from build123d import *

# Parameters (mm, degrees)
SKETCH1_W           = 25.4
SKETCH1_H           = 21.082
BOSS_EXTRUDE1_DEPTH = 27.178
SKETCH2_R           = 2.921
CUT_EXTRUDE1_DEPTH  = 8.5598
SKETCH3_R           = 2.6924
CUT_EXTRUDE2_DEPTH  = 37.665847979
SKETCH9_R           = 1.9558
CUT_EXTRUDE4_DEPTH  = 27.178
CUT_EXTRUDE3_DEPTH  = 5.08
CUT_EXTRUDE5_START  = -7.62
CUT_EXTRUDE5_DEPTH  = 1.4478
FILLET1_R           = 1.397
FILLET2_R           = 0.635


with BuildPart() as part:
    # Sketch1 → Boss-Extrude1 (new body)
    with BuildSketch(Plane(origin=(0, 0, 0), x_dir=(1, 0, 0), z_dir=(0, 1, 0))):
        Rectangle(SKETCH1_W, SKETCH1_H)
    extrude(amount=BOSS_EXTRUDE1_DEPTH)

    # Sketch2 → Cut-Extrude1 (cut)
    with BuildSketch(Plane(origin=(0, 27.178, 0), x_dir=(1, 0, 0), z_dir=(0, 1, 0))):
        with Locations(Location((-8.128, -4.953, 0), (0, 0, 270))):
            Circle(SKETCH2_R)
        with Locations(Location((-8.128, 4.953, 0), (0, 0, 270))):
            Circle(SKETCH2_R)
    extrude(amount=-CUT_EXTRUDE1_DEPTH, mode=Mode.SUBTRACT)

    # Sketch3 → Cut-Extrude2 (cut, through all)
    with BuildSketch(Plane.XY.offset(10.541)):
        with Locations((3.81, 13.589)):
            Circle(SKETCH3_R)
    extrude(amount=-CUT_EXTRUDE2_DEPTH, mode=Mode.SUBTRACT)

    # Sketch9 → Cut-Extrude4 (cut)
    with BuildSketch(Plane(origin=(0, 27.178, 0), x_dir=(1, 0, 0), z_dir=(0, 1, 0))):
        with Locations(Location((-8.128, 4.953, 0), (0, 0, 270))):
            Circle(SKETCH9_R)
        with Locations(Location((-8.128, -4.953, 0), (0, 0, 270))):
            Circle(SKETCH9_R)
    extrude(amount=-CUT_EXTRUDE4_DEPTH, mode=Mode.SUBTRACT)

    # Sketch5 → Cut-Extrude3 (cut)
    with BuildSketch(Plane.ZY.offset(12.7)):
        with BuildLine():
            Line((-6.303, 11.494), (-6.303, 0))
            Line((-6.303, 0), (6.397, 0))
            Line((6.397, 0), (6.397, 11.494))
            ThreePointArc((6.397, 11.494), (0.047, 17.844), (-6.303, 11.494))
        make_face()
    extrude(amount=-CUT_EXTRUDE3_DEPTH, mode=Mode.SUBTRACT)

    # Cut-Extrude5: read off the stored shape, not the designer's step
    # Cut-Extrude5 outline → Cut-Extrude5 (cut)
    with BuildSketch(Plane.YZ.offset(CUT_EXTRUDE5_START)):
        with BuildLine():
            Line((15.525583312, 4.953), (0, 4.953))
            Line((0, 4.953), (0, -4.953))
            Line((0, -4.953), (15.408396505, -4.953))
            ThreePointArc((15.408396505, -4.953), (17.843555718, -0.028114492), (15.525583312, 4.953))
        make_face()
    extrude(amount=CUT_EXTRUDE5_DEPTH, mode=Mode.SUBTRACT)

    # Fillet1
    fillet1_edges = [part.edges().sort_by_distance(p)[0] for p in [
        (-12.7, 0, 8.469),
        (0, 0, 10.541),
        (-12.7, 0, -8.422),
        (0, 0, -10.541),
        (12.7, 0, 0),
        (12.7, 13.589, 10.541),
        (-12.7, 13.589, 10.541),
        (-12.7, 13.589, -10.541),
        (12.7, 13.589, -10.541),
    ]]
    fillet(fillet1_edges, radius=FILLET1_R)

    # Fillet2
    fillet2_edges = [part.edges().sort_by_distance(p)[0] for p in [
        (-7.400882257, 0, -6.768613788),
        (-10.375048641, 0, 6.397),
        (-10.423075727, 0, -6.303),
        (-12.7, 17.844, 0.047),
        (-12.7, 6.4455, -6.303),
        (-6.745040557, 0, 6.335959443),
        (-6.1722, 0, 0),
        (-12.7, 6.4455, 6.397),
        (-12.290828173, 0.409171827, -6.303),
        (-12.290828173, 0.409171827, 6.397),
    ]]
    fillet(fillet2_edges, radius=FILLET2_R)


solid = part.part
The model under review builds one solid part; all positions refer to its coordinate system, in mm. A direction names the side the tool comes from. Coordinates: 2 decimals unless noted, no trailing zeros. Write each loop counter-clockwise with the first axis right and the second up, starting at its lowest first coordinate (ties: lowest second). Pieces come first, ordered by that corner, then holes. Notation, with made-up numbers: (72, -36) - (128, -36) arc R15 cw to (128, -21) - close; hole circle Ø4 at (-17.5, -8.5). An arc over 180 degrees is marked (long way). Answer as a JSON object with one key per item and string values. Group by question number.
1. Mouldability with a two-part tool opening along Z and no side actions: class faces 1 (the face through (12.28, 14.47, 10.14)), 2 (the face through (-5.232, 22.958, 4.573)), 3 (the face through (0, 27.178, 0)), 4 (the face through (-7.251, 22.958, -2.167)) as pulls with the +Z half, pulls with the -Z half, needs draft (parallel to the pull), parting line crosses it, or undercut.
2. To check wall thickness, follow probe 1 along Z at (x, y) = (-9.75, 4.25); probe 2 along Z at (x, y) = (-8, 2.75); probe 3 along X at (y, z) = (6, -3). State the ranges of each line that lie inside material, in increasing order.
3. Machinability: for faces 5 (the face through (-11, 6, 6.397)), 6 (the face through (-10, 18.618, 6)), 7 (the face through (6.378, 14.398, 0.148)), which of the approach directions +Z, -Z, +X, -X, +Y, -Y give a long, thin tool a straight path to every point of the face, cutting with its end or side? Answer none if there is none.
4. Add section A-A (x = 3.81). Give the boundary of the cut face in (y, z).
5. Add section B-B (y = 8.75). Give the boundary of the cut face in (x, z) (3 decimals).
6. Clearance check with flat-ended pins moving along their axes: pin 1 Ø1.8 at (x, z) = (-9, -6.5) entering from +Y; pin 2 Ø5 at (y, z) = (8, -2) entering from -X. State where each tip first meets the part, or that it passes through.
7. Add section C-C (y = 21). Give the boundary of the cut face in (x, z).
8. Add section D-D (z = -5.5). Give the number of separate pieces and of enclosed holes in the cut face, plus the area to 3 significant figures.
Findings:
{
 "1": {"face 1": "pulls with the +Z half", "face 2": "undercut", "face 3": "needs draft", "face 4": "undercut"},
 "2": {"probe 1": "-10.54 to -6.3, 6.4 to 10.54", "probe 2": "-10.54 to -6.9, 6.9 to 10.54", "probe 3": "-6.17 to 12.7"},
 "3": {"face 5": "-X, -Y", "face 6": "+Y", "face 7": "+Z, -Z"},
 "4": {"outline": "(0, -9.14) arc R1.4 ccw to (1.4, -10.54) - (10.9, -10.54) - (10.9, 10.54) - (1.4, 10.54) arc R1.4 ccw to (0, 9.14) - close; (16.28, -10.54) - (27.18, -10.54) - (27.18, 10.54) - (16.28, 10.54) - close"},
 "5": {"outline": "(-12.7, -9.144) arc R1.397 ccw to (-11.303, -10.541) - (11.303, -10.541) arc R1.397 ccw to (12.7, -9.144) - (12.7, 9.144) arc R1.397 ccw to (11.303, 10.541) - (-11.303, 10.541) arc R1.397 ccw to (-12.7, 9.144) - (-12.7, 7.032) arc R0.635 ccw to (-12.065, 6.397) - (-9.447, 6.397) arc R1.956 cw to (-6.172, 4.953) - (-6.172, -4.953) arc R1.956 cw to (-9.543, -6.303) - (-12.065, -6.303) arc R0.635 ccw to (-12.7, -6.938) - close"},
 "6": {"pin 1": "y = 18.62", "pin 2": "x = -6.17"},
 "7": {"outline": "(-12.7, -9.14) arc R1.4 ccw to (-11.3, -10.54) - (11.3, -10.54) arc R1.4 ccw to (12.7, -9.14) - (12.7, 9.14) arc R1.4 ccw to (11.3, 10.54) - (-11.3, 10.54) arc R1.4 ccw to (-12.7, 9.14) - close; hole circle Ø5.84 at (-8.13, -4.95); hole circle Ø5.84 at (-8.13, 4.95)"},
 "8": {"separate pieces": "2", "enclosed holes": "1", "area": "509 mm²"}
}
